Geometry: see drawing. Coordinates: mm, zero at the bounding-box minimum. A direction names the side the tool comes from. Give positions to 0.01 mm unless a question says otherwise; leave off trailing zeros. Order: outer loops, then holes, each group sorted by start corner. A loop starts at its lowest first (then second) coordinate and runs counter-clockwise, first axis right, second up. Notation, with made-up numbers: (12.5, 84) - (58.5, 84) arc R8 ccw to (58.5, 94) - close; hole circle Ø6 at (12.25, 52). An arc over 180 degrees is marked (long way). Write each question's results on one line, items separated by ' | '. Start each with the question number.
Item 1: Mould query, pull axis X, two halves, no side actions, for the marked faces 3, 4 and 5. Classes: released by +X, released by -X, zero draft, split by the parting line, or undercut.
Item 2: Section A-A on x = 31.5. Output: boundary loops of the cut face in (y, z), and give its area (3 significant figures).
Item 3: Line query: line 1 along Z through (x, y) = (10, 33); line 2 along X through (y, z) = (37, 6.5) (1 decimal); line 3 along Y through (x, z) = (35, 6.95). Output: solid intervals per line, ascending.
Item 4: Section D-D on x = 4. Output: boundary loops of the cut face in (y, z).
Item 5: Set-up query: the marked faces 1 and 2. Return all of +Z, -Z, +X, -X, +Y, -Y with unobstructed straight access to the full face (end or side cutting, diameter ignored); none if empty.
Item 6: Section B-B on z = 3.5. Output: boundary loops of the cut face in (x, y).
Item 7: Contact query for flat-ended pins moving along their axis: pin 1 Ø2 at (y, z) = (35.5, 6) entering from +X; pin 2 Ø1.5 at (y, z) = (39, 4.5) entering from -X; pin 3 Ø1.5 at (x, z) = (9, 5) entering from +Y; pin 4 Ø4 at (x, y) = (5, 39.24) entering from -Z. Output: stop coordinate, or through.
Item 8: Section C-C on x = 35.5. Output: boundary loops of the cut face in (y, z), and give its area (3 significant figures).
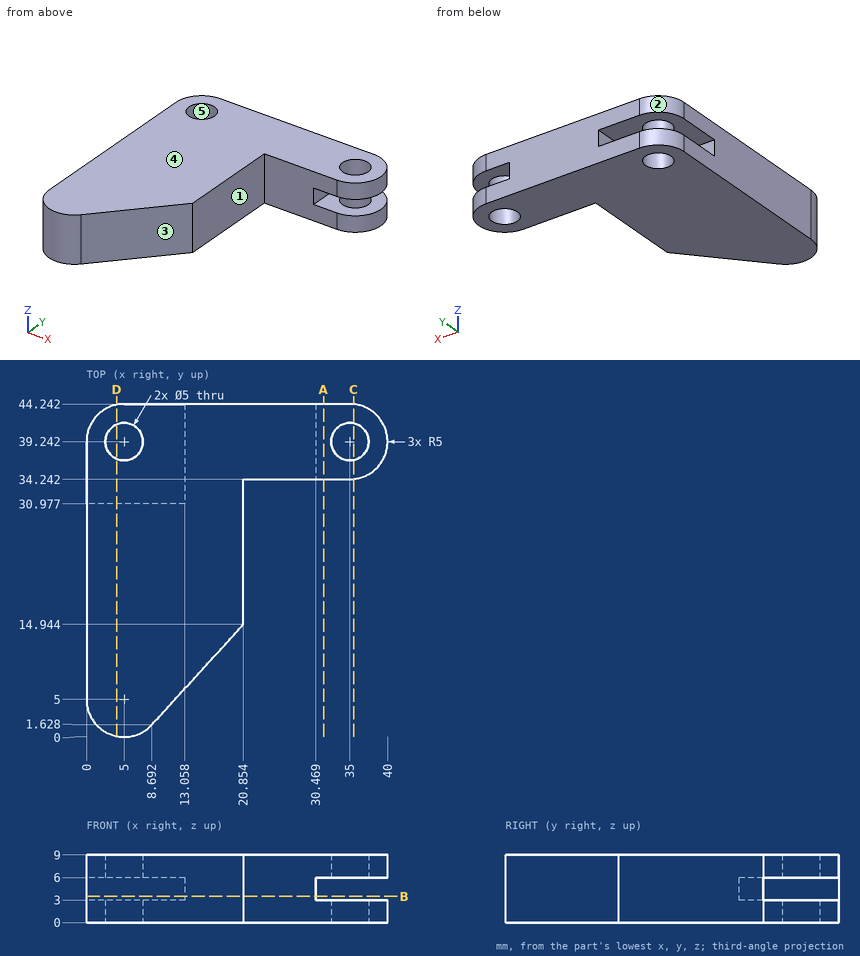
Evaluation:
1) face 3: released by +X | face 4: zero draft | face 5: undercut
2) outline: (34.24, 0) - (44.24, 0) - (44.24, 3) - (34.24, 3) - close; (34.24, 6) - (44.24, 6) - (44.24, 9) - (34.24, 9) - close | area: 60.0 mm^2
3) line 1: z = 0 to 3, 6 to 9 | line 2: x = 0 to 3.9, 6.1 to 33.9, 36.1 to 39.5 | line 3: y = 34.24 to 36.74, 41.74 to 44.24
4) outline: (0.1, 0) - (36.95, 0) - (36.95, 3) - (30.98, 3) - (30.98, 6) - (36.95, 6) - (36.95, 9) - (0.1, 9) - close; (41.53, 0) - (44.14, 0) - (44.14, 3) - (41.53, 3) - close; (41.53, 6) - (44.14, 6) - (44.14, 9) - (41.53, 9) - close
5) face 1: +Z, -Z, +X, -Y | face 2: +Z, -Z, -X, +Y
6) outline: (0, 5) arc R5 ccw to (8.69, 1.63) - (20.85, 14.94) - (20.85, 34.24) - (30.47, 34.24) - (30.47, 44.24) - (13.06, 44.24) - (13.06, 30.98) - (0, 30.98) - close
7) pin 1: stops at x = 39.18 | pin 2: stops at x = 13.06 | pin 3: stops at y = 30.98 | pin 4: passes through
8) outline: (34.27, 0) - (36.79, 0) - (36.79, 3) - (34.27, 3) - close; (34.27, 6) - (36.79, 6) - (36.79, 9) - (34.27, 9) - close; (41.69, 0) - (44.22, 0) - (44.22, 3) - (41.69, 3) - close; (41.69, 6) - (44.22, 6) - (44.22, 9) - (41.69, 9) - close | area: 30.3 mm^2
